The model under review builds one solid part; all positions refer to its coordinate system, in mm. Coordinates: 2 decimals unless noted, no trailing zeros. Order: outer loops, then holes, each group sorted by start corner. A loop starts at its lowest first (then second) coordinate and runs counter-clockwise, first axis right, second up.
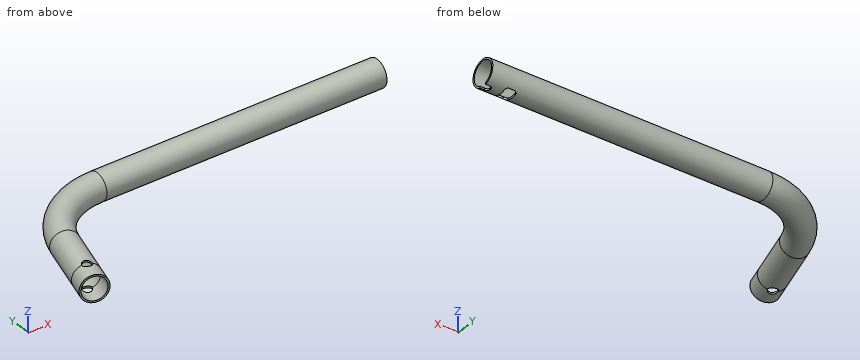
```python
from build123d import *

# Parameters (mm, degrees)
SKETCH3_R          = 9.5
SKETCH3_R_2        = 8.3
CUT_EXTRUDE1_REACH = 191.877
SKETCH4_R          = 3.3
SKETCH5_R          = 3.3
CUT_EXTRUDE2_DEPTH = 190.876682823


with BuildPart() as part:
    # Sweep2: sweep along a path in Sketch1
    with BuildLine(Plane.XY) as sweep2_path:
        Line((108.839588828, 0), (92.239588828, 0))
        Line((92.239588828, 0), (-92.239588828, 0))
        ThreePointArc((-92.239588828, 0), (-124.360019313, -10.591729527), (-143.88004565, -38.211927945))
        Line((-143.88004565, -38.211927945), (-154.760411172, -73.8))
        Line((-154.760411172, -73.8), (-158.490325485, -86))
    # Sketch3 → Sweep2 (sweep)
    with BuildSketch(Plane(origin=(92.239588828, 0, 0), x_dir=(0, 0, -1), z_dir=(1, 0, 0))):
        Circle(SKETCH3_R)
        Circle(SKETCH3_R_2, mode=Mode.SUBTRACT)
    sweep(path=sweep2_path.line)

    # Sketch4 → Cut-Extrude1 (cut, up to next)
    with BuildSketch(Plane.XY, mode=Mode.PRIVATE) as cut_extrude1_sk1:
        with Locations(Location((-154.760411172, -73.8, 0), (0, 0, 343))):
            Circle(SKETCH4_R)
    cut_extrude1_tool1 = extrude(cut_extrude1_sk1.sketch, amount=-CUT_EXTRUDE1_REACH, mode=Mode.PRIVATE) & part.part
    # Sketch4 → Cut-Extrude1 (cut, up to next)
    with BuildSketch(Plane.XY, mode=Mode.PRIVATE) as cut_extrude1_sk2:
        with BuildLine():
            Line((108.839588828, 2.555545653), (108.839588828, -2.555545653))
            Line((108.839588828, -2.555545653), (105.639588828, -2.555545653))
            ThreePointArc((105.639588828, -2.555545653), (104.225375266, -1.969759216), (103.639588828, -0.555545653))
            Line((103.639588828, -0.555545653), (103.639588828, 0.555545653))
            ThreePointArc((103.639588828, 0.555545653), (104.225375266, 1.969759216), (105.639588828, 2.555545653))
            Line((105.639588828, 2.555545653), (108.839588828, 2.555545653))
        make_face()
    cut_extrude1_tool2 = extrude(cut_extrude1_sk2.sketch, amount=-CUT_EXTRUDE1_REACH, mode=Mode.PRIVATE) & part.part
    # Sketch4 → Cut-Extrude1 (cut, up to next)
    with BuildSketch(Plane.XY, mode=Mode.PRIVATE) as cut_extrude1_sk3:
        with BuildLine():
            Line((90.239588828, -5.5), (94.239588828, -5.5))
            ThreePointArc((94.239588828, -5.5), (95.653802391, -4.914213562), (96.239588828, -3.5))
            Line((96.239588828, -3.5), (96.239588828, 3.5))
            ThreePointArc((96.239588828, 3.5), (95.653802391, 4.914213562), (94.239588828, 5.5))
            Line((94.239588828, 5.5), (90.239588828, 5.5))
            ThreePointArc((90.239588828, 5.5), (88.825375266, 4.914213562), (88.239588828, 3.5))
            Line((88.239588828, 3.5), (88.239588828, -3.5))
            ThreePointArc((88.239588828, -3.5), (88.825375266, -4.914213562), (90.239588828, -5.5))
        make_face()
    cut_extrude1_tool3 = extrude(cut_extrude1_sk3.sketch, amount=-CUT_EXTRUDE1_REACH, mode=Mode.PRIVATE) & part.part
    add(cut_extrude1_tool1.solids().sort_by_distance((-154.760411, -73.8, 0))[0], mode=Mode.SUBTRACT)
    add(cut_extrude1_tool2.solids().sort_by_distance((106.388287, 0, 0))[0], mode=Mode.SUBTRACT)
    add(cut_extrude1_tool3.solids().sort_by_distance((92.239589, 0, 0))[0], mode=Mode.SUBTRACT)

    # Sketch5 → Cut-Extrude2 (cut, through all)
    with BuildSketch(Plane.XY):
        with Locations(Location((-154.760411172, -73.8, 0), (0, 0, 343))):
            Circle(SKETCH5_R)
    extrude(amount=CUT_EXTRUDE2_DEPTH, mode=Mode.SUBTRACT)


solid = part.part
```
(1) We need section A-A, the plane z = 1.5. Write out the cut boundary in (x, y).
A:
outline: (-167.46, -83.26) - (-166.3, -83.61) - (-151.69, -35.83) arc R62.16 cw to (-92.24, 8.16) - (108.84, 8.16) - (108.84, 9.38) - (-92.24, 9.38) arc R63.38 ccw to (-152.85, -35.47) - close; (-150.68, -88.39) - (-149.52, -88.74) - (-134.91, -40.95) arc R44.62 cw to (-92.24, -9.38) - (108.84, -9.38) - (108.84, -8.16) - (-92.24, -8.16) arc R45.84 ccw to (-136.07, -40.6) - close
(2) We need section B-B, the plane x = 57.5. Write out the cut boundary in (y, z).
A:
outline: circle Ø19 at (0, 0); hole circle Ø16.6 at (0, 0)
(3) For pin 1 Ø6 at (x, y) = (-154.76, -73.8) entering from -Z; pin 2 Ø8 at (y, z) = (-78.5, -5.5) entering from +X; pin 3 Ø1.4 at (x, z) = (107, -8) entering from +Y; pin 4 Ø4 at (x, z) = (-126, 7.5) entering from +Y, all flat-tipped, find the tip position at first contact; note any pin that passes through.
A:
pin 1: passes through
pin 2: stops at x = -145.8
pin 3: stops at y = 6.08
pin 4: stops at y = -1.89
(4) Wall thickness on probe 1 along Z at (x, y) = (0, 0.5); probe 2 along Y at (x, z) = (46, 0); probe 3 along X at (y, z) = (-73.8, 8.5): over which ranges is each line inside the solid? List them lowest first.
A:
probe 1: z = -9.49 to -8.28, 8.28 to 9.49
probe 2: y = -9.5 to -8.3, 8.3 to 9.5
probe 3: x = -159.2 to -158.06, -151.46 to -150.32
